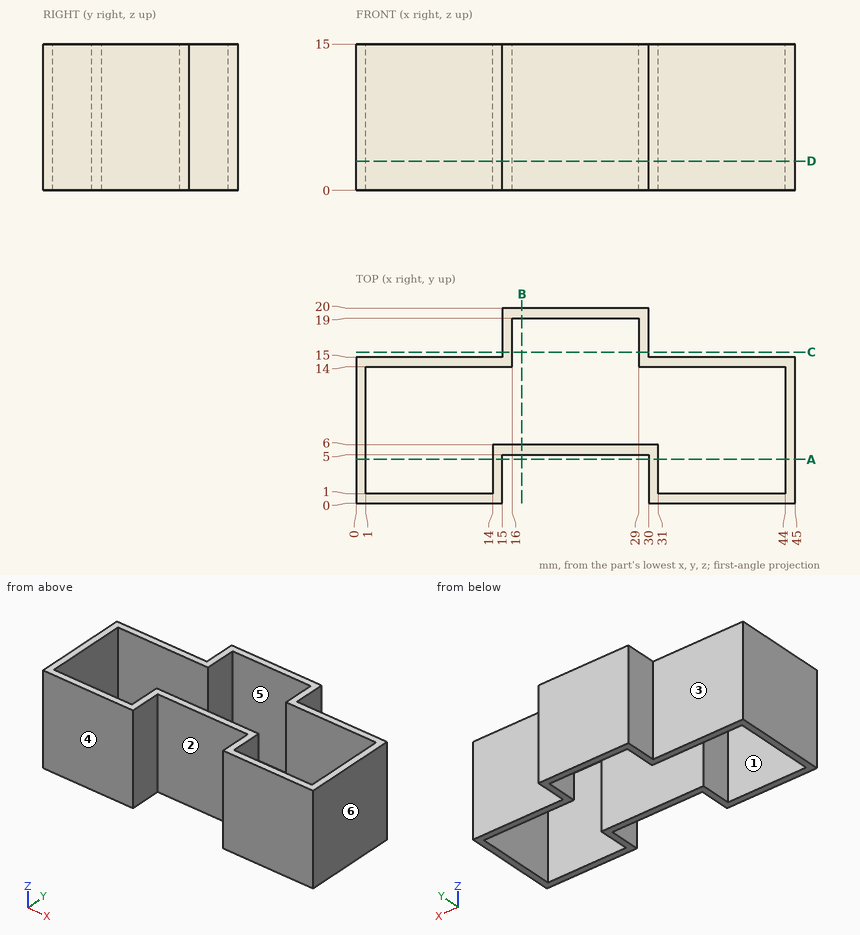
Input: dimensioned drawing with shaded views. Units: mm. Origin: part minimum x, y, z. A direction names the side the tool comes from. Round coordinates to 2 decimals unless told otherwise and drop trailing zeros. Loops run counter-clockwise (first coordinate to the right, second up) from the corner with the lowest first, then second, coordinate; pieces in that order, holes last. Notation, with made-up numbers: (41, 0) -> (96, 0) arc R20 cw to (96, 21) -> close; hole circle Ø3 at (-20, 80). An arc over 180 degrees is marked (long way). Answer as a JSON object with one key per item and string values. Group by question number.
Q1. Section query D-D (z = 3). Output: boundary loops of the cut face in (x, y).
Q2. Mould query, pull axis Y, two halves, no side actions, for the marked faces 4, 5 and 6. Classes: pulls with the +Y half, pulls with the -Y half, needs draft (parallel to the pull), parting line crosses it, or undercut.
Q3. Ray query, line 1 (X direction, y = 5.5, z = 9); line 2 (X direction, y = 1.5, z = 14.25); line 3 (X direction, y = 17.75, z = 2). Return the intervals inside material, ascending. Write a range as from..to.
Q4. Contact query for flat-ended pins moving along their axis: P1, Ø5, axis at x = 25, z = 11.5, coming from the -Y side; P2, Ø2.5, axis at y = 17.5, z = 5.5, coming from the -X side; P3, Ø2.5, axis at y = 18.5, z = 5, coming from the +X side. Output: stop coordinate, or through.
Q5. Section query A-A (y = 4.5). Output: boundary loops of the cut face in (x, z), plus the area to 3 significant figures.
Q6. Section query B-B (x = 17). Output: boundary loops of the cut face in (y, z).
Q7. Section query C-C (y = 15.5). Output: boundary loops of the cut face in (x, z).
Q8. Access query for the marked faces 1, 2 and 3. Directions: +Z, -Z, +X, -X, +Y, -Y. A direction counts if a zero-diameter tool reaches every point of the face in a straight line with its end or side. Return the directions, or none.
Completed:
{
 "1": {"outline": "(0, 0) -> (15, 0) -> (15, 5) -> (30, 5) -> (30, 0) -> (45, 0) -> (45, 15) -> (30, 15) -> (30, 20) -> (15, 20) -> (15, 15) -> (0, 15) -> close; hole (1, 1) -> (14, 1) -> (14, 6) -> (31, 6) -> (31, 1) -> (44, 1) -> (44, 14) -> (29, 14) -> (29, 19) -> (16, 19) -> (16, 14) -> (1, 14) -> close"},
 "2": {"face 4": "pulls with the -Y half", "face 5": "undercut", "face 6": "needs draft"},
 "3": {"line 1": "0..1, 14..31, 44..45", "line 2": "0..1, 14..15, 30..31, 44..45", "line 3": "15..16, 29..30"},
 "4": {"P1": "y = 5", "P2": "x = 15", "P3": "x = 30"},
 "5": {"outline": "(0, 0) -> (1, 0) -> (1, 15) -> (0, 15) -> close; (14, 0) -> (15, 0) -> (15, 15) -> (14, 15) -> close; (30, 0) -> (31, 0) -> (31, 15) -> (30, 15) -> close; (44, 0) -> (45, 0) -> (45, 15) -> (44, 15) -> close", "area": "60.0 mm²"},
 "6": {"outline": "(5, 0) -> (6, 0) -> (6, 15) -> (5, 15) -> close; (19, 0) -> (20, 0) -> (20, 15) -> (19, 15) -> close"},
 "7": {"outline": "(15, 0) -> (16, 0) -> (16, 15) -> (15, 15) -> close; (29, 0) -> (30, 0) -> (30, 15) -> (29, 15) -> close"},
 "8": {"face 1": "+Z, -Z", "face 2": "+Z, -Z, -Y", "face 3": "+Z, -Z, -X, +Y"}
}
